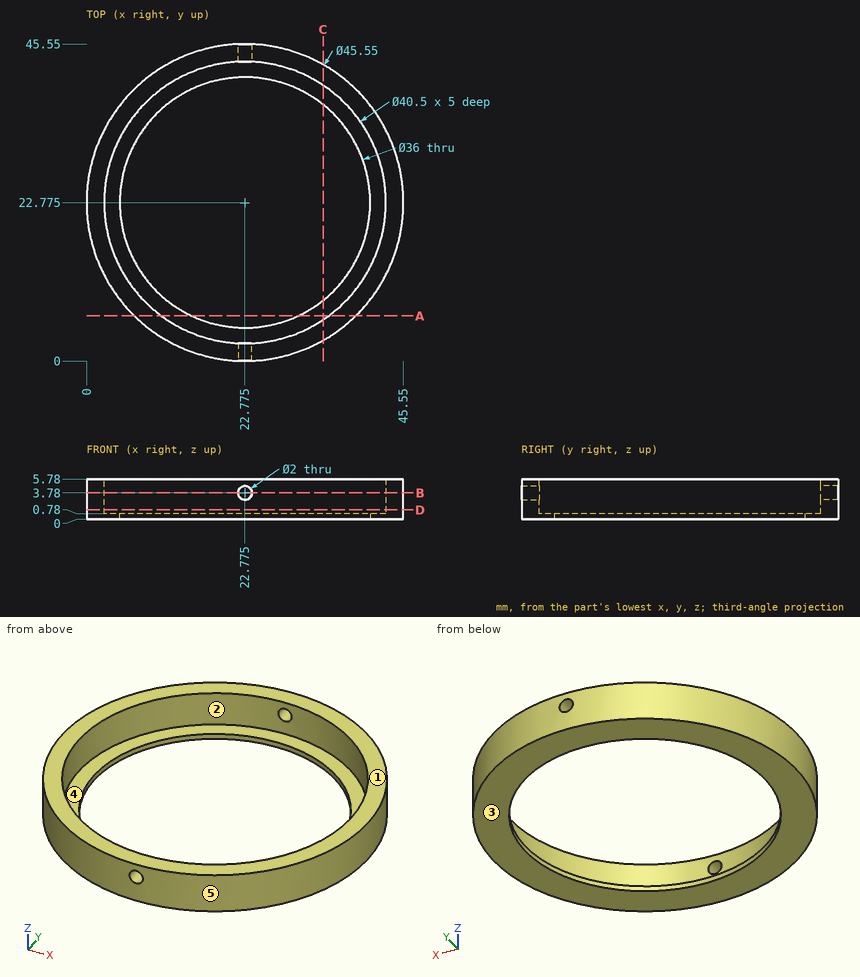
Input: dimensioned drawing with shaded views. Units: mm. Origin: part minimum x, y, z. A direction names the side the tool comes from. Give positions to 0.01 mm unless a question says otherwise; leave off trailing zeros. Write each loop counter-clockwise with the first axis right and the second up, starting at its lowest first coordinate (ties: lowest second). Pieces come first, ordered by that corner, then holes.
1. Section query A-A, the plane y = 6.5. Return loops of the section in (x, z).
2. Draft query along X for the marked faces 3, 4 and 5. Return one class per face: released by +X, released by -X, zero draft, split by the parting line, or undercut.
3. Section query C-C, the plane x = 34. Return loops of the section in (y, z).
4. Section query B-B, the plane z = 3.78. Return loops of the section in (x, y) (3 decimals), then the cut area to 3 significant figures.
5. Line query: probe 1 along Z at (x, y) = (42.5, 26); probe 2 along Y at (x, z) = (41, 0.95); probe 3 along X at (y, z) = (29.5, 1.75). Output: solid intervals per line, ascending.
6. Pin query (flat end, axial travel): P1, Ø3, axis at x = 31, z = 2.5, coming from the -Y side; P2, Ø2, axis at x = 15.5, z = 1.5, coming from the -Y side; P3, Ø1, axis at x = 14.5, z = 2, coming from the -Y side. Return the tip coordinate at first contact, or that it passes through.
7. Reachability of the marked faces 1 and 2 from +Z, -Z, +X, -X, +Y, -Y: full face, straight path, thin tool, end or side. Return the list, or none.
8. Section query D-D, the plane z = 1.35. Return loops of the section in (x, y) (3 decimals).
Computed:
1. outline: (6.84, 0) - (15.09, 0) - (15.09, 0.78) - (10.73, 0.78) - (10.73, 5.78) - (6.84, 5.78) - close; (30.46, 0) - (38.71, 0) - (38.71, 5.78) - (34.82, 5.78) - (34.82, 0.78) - (30.46, 0.78) - close
2. face 3: zero draft
2. face 4: undercut
2. face 5: split by the parting line
3. outline: (2.96, 0) - (8.7, 0) - (8.7, 0.78) - (5.92, 0.78) - (5.92, 5.78) - (2.96, 5.78) - close; (36.85, 0) - (42.59, 0) - (42.59, 5.78) - (39.63, 5.78) - (39.63, 0.78) - (36.85, 0.78) - close
4. outline: (21.775, 0.022) - (21.775, 2.55) arc R20.25 cw to (21.775, 43) - (21.775, 45.528) arc R22.775 ccw to start; (23.775, 0.022) arc R22.775 ccw to (23.775, 45.528) - (23.775, 43) arc R20.25 cw to (23.775, 2.55) - close
4. area: 331 mm2
5. probe 1: z = 0 to 0.78
5. probe 2: y = 9.12 to 13.95, 31.6 to 36.43
5. probe 3: x = 1.02 to 3.67, 41.88 to 44.53
6. P1: stops at y = 1.02
6. P2: stops at y = 0.88
6. P3: stops at y = 1.37
7. face 1: +Z, +X, -X, +Y, -Y
7. face 2: +Z
8. outline: circle Ø45.55 at (22.775, 22.775); hole circle Ø40.5 at (22.775, 22.775)
